The listing builds one solid part. Answer for the finished solid, in the listing's coordinates (mm). Round coordinates to 2 decimals unless told otherwise and drop trailing zeros. Loops run counter-clockwise (first coordinate to the right, second up) from the corner with the lowest first, then second, coordinate; pieces in that order, holes last. Notation, with made-up numbers: (87, -19) -> (107, -19) arc R27 ccw to (107, 18) -> close; hole circle Ø8 at (-23.5, -4.75). An arc over 180 degrees is marked (long way). One line per question, with ' | ' between items.
Autodesk Inventor part; units mm, degrees
ref_plane "YZ Plane" through (0, 0, 0) normal (1, 0, 0) x (0, 1, 0)
ref_plane "XZ Plane" through (0, 0, 0) normal (0, 1, 0) x (-1, 0, 0)
ref_plane "XY Plane" through (0, 0, 0) normal (0, 0, 1) x (1, 0, 0)
sketch "Skizze1" plane through (0, 0, 0) normal (0, 0, 1) x (1, 0, 0)
  line L0 (-3.25, -1.75) -> (3.25, -1.75)
  line L1 (3.25, -1.75) -> (3.25, 1.75)
  line L2 (3.25, 1.75) -> (-3.25, 1.75)
  line L3 (-3.25, 1.75) -> (-3.25, -1.75)
  line L4 (-3.25, -1.75) -> (3.25, 1.75) construction
  line L5 (3.25, -1.75) -> (-3.25, 1.75) construction
  point P0 (0, 0)
  dimension "d0" = 6.5
  dimension "d1" = 3.5
extrude "Extrusion1" add sketch "Skizze1" along normal blind 1.5
sketch "Skizze2" plane through (3.25, -1.75, 0) normal (1, 0, 0) x (0, 0, -1)
  line L0 (0, 3.5) -> (-1.5, 3.5)
  line L1 (-0.7, 3.5) -> (-0.7, 4.0328)
  line L2 (-0.7, 4.0328) -> (-0.2, 4.5328)
  line L3 (-0.2, 4.5328) -> (-0.2, 5.25)
  line L4 (-0.2, 5.25) -> (0, 5.25)
  line L5 (0, 5.25) -> (0, 4.45)
  line L6 (0, 4.45) -> (-0.5, 3.95)
  line L7 (-0.5, 3.95) -> (-0.5, 3.5)
  line L8 (0, 0) -> (0, 3.5)
  point P0 (0, 1.75)
  dimension "d4" = 0.8
  dimension "d5" = 0.7
  dimension "d6" = 0.2
  dimension "d7" = 0.2
  dimension "d8" = 0.2
  dimension "d9" = 1.75
  dimension "d10" = 45
extrude "Extrusion2" add sketch "Skizze2" against normal blind 6.5
mirror "Spiegeln1" about plane through (0, 0, 0) normal (0, 1, 0) of "Extrusion2"
sketch "Skizze3" plane through (0, 0, 1.5) normal (0, 0, 1) x (1, 0, 0)
  line L0 (-3.25, 3.5) -> (-1.5, 3.5)
  line L1 (-1.5, 3.5) -> (-1.5, 1.75)
  line L2 (-1.5, 1.75) -> (-3.25, 1.75)
  line L3 (-3.25, 1.75) -> (-3.25, 3.5)
  line L4 (1.5, 3.5) -> (3.25, 3.5)
  line L5 (3.25, 3.5) -> (3.25, 1.75)
  line L6 (3.25, 1.75) -> (1.5, 1.75)
  line L7 (1.5, 1.75) -> (1.5, 3.5)
  line L8 (-3.25, -3.5) -> (-2.7, -3.5)
  line L9 (-2.7, -3.5) -> (-2.7, -1.75)
  line L10 (-2.7, -1.75) -> (-3.25, -1.75)
  line L11 (-3.25, -1.75) -> (-3.25, -3.5)
  line L12 (-0.25, -3.5) -> (-2.2, -3.5)
  line L13 (-2.2, -3.5) -> (-2.2, -1.75)
  line L14 (-2.2, -1.75) -> (-0.25, -1.75)
  line L15 (-0.25, -1.75) -> (-0.25, -3.5)
  line L16 (0.25, -1.75) -> (2.2, -1.75)
  line L17 (2.2, -1.75) -> (2.2, -3.5)
  line L18 (2.2, -3.5) -> (0.25, -3.5)
  line L19 (0.25, -3.5) -> (0.25, -1.75)
  line L20 (2.7, -3.5) -> (3.25, -3.5)
  line L21 (3.25, -3.5) -> (3.25, -1.75)
  line L22 (3.25, -1.75) -> (2.7, -1.75)
  line L23 (2.7, -1.75) -> (2.7, -3.5)
  line L24 (-3.25, -1.75) -> (3.25, -1.75)
  line L25 (3.25, 3.5) -> (-3.25, 3.5)
  line L26 (3.25, 1.75) -> (-3.25, 1.75)
  line L27 (3.25, 3.5) -> (3.25, 2.7828)
  line L28 (-3.25, 2.7828) -> (-3.25, 3.5)
  line L29 (0, 5.1518) -> (0, -6.0635) construction
  line L30 (3.25, -2.2828) -> (3.25, -1.75) construction
  line L31 (3.25, -3.5) -> (-3.25, -3.5) construction
  point P0 (0, 0)
  dimension "d13" = 3
  dimension "d14" = 0.5
  dimension "d15" = 5.4
  dimension "d16" = 0.5
extrude "Extrusion3" cut sketch "Skizze3" against normal blind 6.5 contours L0 L1 L2 L3 | L4 L5 L6 L7 | L11 L10 L9 L8 | L22 L21 L20 L23 | L16 L17 L18 L19 | L14 L15 L12 L13
chamfer "Fase1" distance 0.3 distance2 0.8 1 edges at (0, 1.75, 1.5) measured on face at (1.0833, -0.5833, 1.5)
chamfer "Fase2" distance 0.3 distance2 0.8 1 edges at (0, -1.75, 1.5) measured on face at (-1.0833, 0.3837, 1.5)
chamfer "Fase3" distance 0.5 distance2 0.15 1 edges at (0, 1.75, 0) measured on face at (0.5, 1.75, 0.1667)
chamfer "Fase4" distance 0.5 distance2 0.15 1 edges at (0, -1.75, 0) measured on face at (-0.0833, -1.75, 0.1667)
fillet "Rundung1" radius 0.4 16 edges at (2.45, -2.2828, 0.7) (2.45, -2.2, 0.5) (2.45, -2.7, 0) (2.45, -2.7828, 0.2) (0, -2.2, 0.5) (0, -2.7, 0) (0, -2.2828, 0.7) (0, -2.7828, 0.2) (-2.45, -2.2828, 0.7) (-2.45, -2.2, 0.5) (-2.45, -2.7, 0) (-2.45, -2.7828, 0.2) (0, 2.7, 0) (0, 2.7828, 0.2) (0, 2.2, 0.5) (0, 2.2828, 0.7)
chamfer "Fase5" distance 0.5 distance2 0.15 1 edges at (-3.25, 0, 0) measured on face at (-3.25, 0.4835, 0.5)
chamfer "Fase6" distance 0.5 distance2 0.15 1 edges at (3.25, 0, 0) measured on face at (3.25, -0.4835, 0.5)
chamfer "Fase7" distance 0.3 distance2 0.8 1 edges at (3.25, 0, 1.5) measured on face at (-1.0833, 0.4835, 1.5)
chamfer "Fase8" distance 0.3 distance2 0.8 1 edges at (-3.25, 0, 1.5) measured on face at (0.8833, -0.4835, 1.5)
equation "\"d8\" = d7"
properties part number "AMS1117"
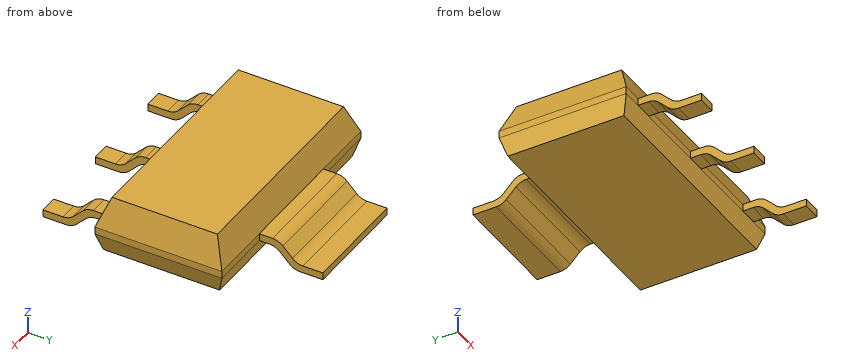
Q1. Find the intervals of material crossed by line 1 (Y direction, x = -1.5, z = 1.1); line 2 (Y direction, x = 1.25, z = 0.3); line 3 (X direction, y = 3, z = 0.1), in increasing order. Write a range as from..to.
Numbers:
line 1: -1.6..1.6 | line 2: -1.69..1.69, 2.4..2.68 | line 3: -1.5..1.5
Q2. Given pin 1 Ø0.6 at (y, z) = (-2.5, 0.5) entering from -X; pin 2 Ø0.8 at (y, z) = (-2.5, 0) entering from +X, each flat-ended and moving along its own axis, determine where each tip first touches the part or whether it passes through.
Numbers:
pin 1: x = -2.7 | pin 2: x = 2.7
Q3. A cutting plane is placed at C-C on y = 0.5. Give the vertices of the cut face in (x, z).
Numbers:
outline: (-3.25, 0.5) -> (-3.1, 0) -> (3.1, 0) -> (3.25, 0.5) -> (3.25, 0.7) -> (2.95, 1.5) -> (-2.95, 1.5) -> (-3.25, 0.7) -> close
Q4. A cutting plane is placed at B-B on y = -2.5. Give the vertices of the cut face in (x, z).
Numbers:
outline: (-2.7, 0.2) -> (-2.2, 0.2) -> (-2.2, 0.48) -> (-2.7, 0.48) -> close; (-0.25, 0.2) -> (0.25, 0.2) -> (0.25, 0.48) -> (-0.25, 0.48) -> close; (2.2, 0.2) -> (2.7, 0.2) -> (2.7, 0.48) -> (2.2, 0.48) -> close
